Geometry: final body of the model. Coordinates: model frame, mm. Give positions to 0.01 mm unless a question says otherwise; leave off trailing zeros. Order: outer loops, then holes, each group sorted by start corner. A loop starts at its lowest first (then second) coordinate and runs counter-clockwise, first axis right, second up. Notation, with made-up numbers: (37.25, -4) - (72.25, -4) arc R29 ccw to (72.25, 33) - close; hole circle Ø3 at (22, -30.75). An arc over 180 degrees is marked (long way). Write item = value, one per line. Start each with the question number.
from build123d import *

# Parameters (mm, degrees)
FILLET2_R        = 0.2
LPATTERN10_COUNT = 20
LPATTERN10_PITCH = 0.25


with BuildPart() as part:
    # Sketch1 → Revolve1 (revolve)
    with BuildSketch(Plane(origin=(0, 0, 0), x_dir=(1, 0, 0), z_dir=(0, 1, 0))):
        with BuildLine():
            Line((2.37, 1.5), (17.37, 1.5))
            Line((17.37, 1.5), (17.37, 0))
            Line((17.37, 0), (0, 0))
            ThreePointArc((0, 0), (0.224879408, 1.215980768), (0.869770135, 2.271109163))
            ThreePointArc((0.869770135, 2.271109163), (1.549177667, 2.754228297), (2.37, 2.9))
            Line((2.37, 2.9), (2.37, 1.5))
        make_face()
    revolve(axis=Axis((-13.629268293, 0, 0), (1, 0, 0)))

    # Fillet2
    fillet2_edges = [part.edges().sort_by_distance(p)[0] for p in [
        (2.37, 0, 1.5),
    ]]
    fillet(fillet2_edges, radius=FILLET2_R)

    # Sketch4 → Cut-Revolve1 (revolve, cut)
    with BuildSketch(Plane(origin=(0, 0, 0), x_dir=(1, 0, 0), z_dir=(0, 1, 0))):
        Polygon((18.103454633, 0), (18.103454633, 21), (11.743066959, 21), (17.37, 0), align=None)
    revolve(axis=Axis((4.782773752, 0, 0), (1, 0, 0)), mode=Mode.SUBTRACT)

    # Sketch2 → Cut-Loft1 section 0
    with BuildSketch(Plane(origin=(0, 0, 0), x_dir=(0, 0, -1), z_dir=(1, 0, 0)), mode=Mode.PRIVATE) as cut_loft1_s0:
        Polygon((-0.4625, 0.4625), (-1.85, 0.4625), (-1.85, -0.4625), (-0.4625, -0.4625), (-0.4625, -1.85), (0.4625, -1.85), (0.4625, -0.4625), (1.85, -0.4625), (1.85, 0.4625), (0.4625, 0.4625), (0.4625, 1.85), (-0.4625, 1.85), align=None)
    loft([Vertex(2.62, 0, 0), cut_loft1_s0.sketch], mode=Mode.SUBTRACT)

    # Sketch6 → Cut-Revolve10 (revolve, cut)
    with BuildSketch(Plane.XY):
        Polygon((12.37, 1.7), (12.495, 1.7), (12.495, 1.5), (12.4325, 1.391746825), (12.37, 1.5), align=None)
    cut_revolve10 = revolve(axis=Axis((10.774329131, 0, 0), (-1, 0, 0)), mode=Mode.SUBTRACT)

    # LPattern10: Cut-Revolve10 ×20
    with Locations(*[(i * LPATTERN10_PITCH, 0, 0) for i in range(1, LPATTERN10_COUNT)]):
        add(cut_revolve10, mode=Mode.SUBTRACT)


solid = part.part
Q1. Material intervals for line 1 along Y through (x, z) = (4, -0.3); line 2 along X through (y, z) = (1.4, -2.4); line 3 along Z through (x, y) = (1.25, -2.2), sorted ascending. Write a range as from..to.
Q2. Section A-A, the plane x = 8.5. Return the cut outline in (y, z).
Q3. Contact query for flat-ended pins moving along their axis: pin 1 (1 mm diameter, centred on y = -1.5, z = 0.5, fed in from +X); pin 2 (2 mm diameter, centred on x = 6, z = -0.5, fed in from -Y); pin 3 (3 mm diameter, centred on x = 14.5, z = 0.5, fed in from +Y); pin 4 (3 mm diameter, centred on y = 0, z = 1, fed in from +X). Output: stop coordinate, or through.
The answers:
q1.line_1 = -1.47..1.47
q1.line_2 = 1.61..2.37
q1.line_3 = -1.38..1.38
q2.outline = circle Ø3 at (0, 0)
q3.pin_1 = 17.08
q3.pin_2 = -1.5
q3.pin_3 = 1.5
q3.pin_4 = 17.37
